For this review, take the finished solid that the model builds, in its own axes (mm). Give positions to 0.01 mm unless a question says otherwise; leave off trailing zeros. Order: outer loops, then holes, each group sorted by start corner. A loop starts at its lowest first (then second) coordinate and runs counter-clockwise, first axis right, second up.
Item 1: Consider section D-D (x = 3.5). Give the boundary of the cut face in (y, z) (3 decimals), plus the area to 3 significant figures.
Item 2: Consider section B-B (y = 0). Give the boundary of the cut face in (x, z) (3 decimals).
Item 3: For P1, Ø1.8, axis at y = 6.35, z = 0, coming from the +X side; P2, Ø2, axis at x = 2, y = -1.5, coming from the -Z side, all flat-tipped, find the tip position at first contact; note any pin that passes through.
Item 4: The part is to be moulded in two halves that separate along Y. For faces 1 (the cylindrical face through (3.22, -0.69, -3.1)), 2 (the flat face through (0, 3, -3)), 3 (the cylindrical face through (5.38, -2.75, -12.4)), say which applies: released by +Y, released by -Y, zero draft, split by the parting line, or undercut.
Item 5: For probe 1 along Y at (x, z) = (2.5, -1); probe 2 along X at (y, z) = (-9.75, 7.25); probe 3 along Z at (x, y) = (3.75, 0) (3 decimals), list the stretches that pass through material, from the lowest coordinate up.
Item 6: Consider section C-C (x = 5). Give the boundary of the cut face in (y, z) (3 decimals), plus the area to 3 significant figures.
Item 7: Consider section A-A (z = 0). Give the boundary of the cut face in (x, y) (3 decimals).
```python
from build123d import *

# Parameters (mm, degrees)
F_3_0MM_DOWEL_HOLE1_D           = 3
F_3_0MM_DOWEL_HOLE1_CSINK_D     = 3.05
F_3_0MM_DOWEL_HOLE1_CSINK_ANGLE = 90


with BuildPart() as part:
    # Sketch1 → Revolve1 (revolve)
    with BuildSketch(Plane.XY):
        with BuildLine():
            Line((0, 3.175), (6.35, 3.175))
            Line((6.35, 3.175), (6.35, 12.7))
            Line((6.35, 12.7), (4.445, 12.7))
            ThreePointArc((4.445, 12.7), (3.175, 11.43), (1.905, 12.7))
            Line((1.905, 12.7), (0, 12.7))
            Line((0, 12.7), (0, 3.175))
        make_face()
    revolve(axis=Axis((0, 0, 0), (1, 0, 0)))

    # Ø3.0mm Dowel Hole1 (through all)
    with Locations(Plane.ZY):
        with Locations((0, 6.35), (0, -6.35)):
            CounterSinkHole(F_3_0MM_DOWEL_HOLE1_D / 2, F_3_0MM_DOWEL_HOLE1_CSINK_D / 2, counter_sink_angle=F_3_0MM_DOWEL_HOLE1_CSINK_ANGLE)


solid = part.part
```
Resolved:
1. outline: circle Ø22.945 at (0, 0); hole circle Ø3 at (-6.35, 0); hole circle Ø6.35 at (0, 0); hole circle Ø3 at (6.35, 0)
1. area: 368 mm2
2. outline: (0, -12.7) - (1.905, -12.7) arc R1.27 cw to (4.445, -12.7) - (6.35, -12.7) - (6.35, -3.175) - (0, -3.175) - close; (0, 3.175) - (6.35, 3.175) - (6.35, 12.7) - (4.445, 12.7) arc R1.27 cw to (1.905, 12.7) - (0, 12.7) - close
3. P1: passes through
3. P2: stops at z = -12.69
4. face 1: undercut
4. face 2: zero draft
4. face 3: split by the parting line
5. probe 1: y = -11.58 to -7.47, -5.23 to -3.01, 3.01 to 5.23, 7.47 to 11.58
5. probe 2: x = 0 to 2.03, 4.32 to 6.35
5. probe 3: z = -11.568 to -3.175, 3.175 to 11.568
6. outline: circle Ø25.4 at (0, 0); hole circle Ø3 at (-6.35, 0); hole circle Ø6.35 at (0, 0); hole circle Ø3 at (6.35, 0)
6. area: 461 mm2
7. outline: (0, -12.7) - (1.905, -12.7) arc R1.27 cw to (4.445, -12.7) - (6.35, -12.7) - (6.35, -7.85) - (0.025, -7.85) - (0, -7.875) - close; (0, -4.825) - (0.025, -4.85) - (6.35, -4.85) - (6.35, -3.175) - (0, -3.175) - close; (0, 3.175) - (6.35, 3.175) - (6.35, 4.85) - (0.025, 4.85) - (0, 4.825) - close; (0, 7.875) - (0.025, 7.85) - (6.35, 7.85) - (6.35, 12.7) - (4.445, 12.7) arc R1.27 cw to (1.905, 12.7) - (0, 12.7) - close
